The model under review builds one solid part; all positions refer to its coordinate system, in mm. A direction names the side the tool comes from. Round coordinates to 2 decimals unless told otherwise and drop trailing zeros. Order: outer loops, then holes, each group sorted by start corner. A loop starts at its lowest first (then second) coordinate and runs counter-clockwise, first axis right, second up. Notation, with made-up numbers: (73.25, 4) -> (97.25, 4) arc R27 cw to (97.25, 31) -> close; hole circle Ø9 at (-39.5, 10). An arc over 180 degrees is marked (long way). Use a Markdown table: item, result. Add a question column.
```python
from build123d import *

# Parameters (mm, degrees)
F0_W         = 34.544
F0_H         = 34.544
F1_DEPTH     = 38.1
F3_R         = 15.748
F4_R         = 2.286
F5_DEPTH     = 34.545
F6_R         = 4.445
F7_DEPTH     = 27.94
F8_S5_R      = 4.445
F8_T6_DEPTH  = 8
F8_S11_R     = 4.445
F8_T12_DEPTH = 8
F9_DEPTH     = 16.51
F2_R         = 8.4455
F10_DEPTH    = 33.782
F10_TAPER    = 0.8
F11_R        = 2.54
F12_R        = 3.81
F13_R        = 5.08
F15_DEPTH    = 38.101


# Not quite as in the source:
# - a fillet or chamfer that OpenCascade refuses, or shapes differently, is made with other operations: its cross-section is extruded or revolved along the edge and cut away or added


with BuildPart() as f1:
    # F0 (on Top) → F1 (new body)
    with BuildSketch(Plane.XY):
        with Locations((17.272, -17.272)):
            Rectangle(F0_W, F0_H)
    extrude(amount=F1_DEPTH)

    # F3
    f3_edges = [f1.edges().sort_by_distance(p)[0] for p in [
        (34.544, -34.544, 19.05),
        (34.544, 0, 19.05),
    ]]
    fillet(f3_edges, radius=F3_R)

    # F4 (on face) → F5 (cut, through all)
    with BuildSketch(Plane(origin=(0, 0, 0), x_dir=(0, -1, 0), z_dir=(-1, 0, 0))):
        with Locations((17.272, 10.16)):
            Circle(F4_R)
        with Locations((17.272, 27.94)):
            Circle(F4_R)
    extrude(amount=-F5_DEPTH, mode=Mode.SUBTRACT)

    # F6 (on face) → F7 (cut)
    with BuildSketch(Plane.YZ.offset(34.544)):
        with Locations((-17.272, 27.94)):
            Circle(F6_R)
        with Locations((-17.272, 10.16)):
            Circle(F6_R)
    extrude(amount=-F7_DEPTH, mode=Mode.SUBTRACT)

    # F8: chamfer of 2.54 on 2 edges, made by hand


with BuildPart() as f8_tool2:
    # F8_s3 → F8_t4 (revolve)
    with BuildSketch(Plane.XY.offset(27.94)):
        Polygon((4.064, -19.558), (6.604, -22.098), (6.604, -19.558), align=None)
    revolve(axis=Axis((6.604, -17.272, 27.94), (-1, 0, 0)))

    # F8_s5 → F8_t6 (intersect, symmetric)
    with BuildSketch(Plane.YZ.offset(5.3)):
        with Locations((-17.272, 27.94)):
            Circle(F8_S5_R)
    extrude(amount=F8_T6_DEPTH, both=True, mode=Mode.INTERSECT)


with BuildPart() as f1_1:
    add(f1.part)

    # F8_t1: cut F8_tool2
    add(f8_tool2.part, mode=Mode.SUBTRACT)


with BuildPart() as f8_tool8:
    # F8_s9 → F8_t10 (revolve)
    with BuildSketch(Plane.XY.offset(10.16)):
        Polygon((4.064, -19.558), (6.604, -22.098), (6.604, -19.558), align=None)
    revolve(axis=Axis((6.604, -17.272, 10.16), (-1, 0, 0)))

    # F8_s11 → F8_t12 (intersect, symmetric)
    with BuildSketch(Plane.YZ.offset(5.3)):
        with Locations((-17.272, 10.16)):
            Circle(F8_S11_R)
    extrude(amount=F8_T12_DEPTH, both=True, mode=Mode.INTERSECT)


with BuildPart() as f1_2:
    add(f1_1.part)

    # F8_t7: cut F8_tool8
    add(f8_tool8.part, mode=Mode.SUBTRACT)

    # F9 (add): a face of the model
    f9_faces = [f1_2.faces().sort_by_distance(p)[0] for p in [
        (0, -17.272, 19.05),
    ]]
    extrude(f9_faces, amount=F9_DEPTH)

    # F2 (on face) → F10 (join)
    with BuildSketch(Plane.XY.offset(38.1)):
        with Locations((17.272, -17.272)):
            Circle(F2_R)
    extrude(amount=F10_DEPTH, taper=F10_TAPER)

    # F11
    f11_edges = [f1_2.edges().sort_by_distance(p)[0] for p in [
        (1.143, 0, 38.1),
        (-16.51, -17.272, 38.1),
        (29.931518, -4.612482, 38.1),
        (1.143, -34.544, 38.1),
        (34.544, -17.272, 38.1),
        (29.931518, -29.931518, 38.1),
        (8.8265, -17.272, 38.1),
    ]]
    fillet(f11_edges, radius=F11_R)

    # F12
    f12_edges = [f1_2.edges().sort_by_distance(p)[0] for p in [
        (1.143, 0, 0),
        (-16.51, -17.272, 0),
        (1.143, -34.544, 0),
        (29.931518, -29.931518, 0),
        (34.544, -17.272, 0),
        (29.931518, -4.612482, 0),
    ]]
    fillet(f12_edges, radius=F12_R)

    # F13
    f13_edges = [f1_2.edges().sort_by_distance(p)[0] for p in [
        (9.298216, -17.272, 71.882),
    ]]
    fillet(f13_edges, radius=F13_R)

    # F14 (on face) → F15 (cut, through all)
    with BuildSketch(Plane.XY.offset(38.1)):
        with BuildLine():
            ThreePointArc((-6.6983271655, -3.81), (-8.9482084501, -5.1711725294), (-8.7866908377, -7.7957998383))
            Line((-8.7866908377, -7.7957998383), (-5.8592190016, -12.0243421801))
            ThreePointArc((-5.8592190016, -12.0243421801), (-3.7708553294, -13.1185423418), (-1.6824916571, -12.0243421801))
            Line((-1.6824916571, -12.0243421801), (1.244980179, -7.7957998383))
            ThreePointArc((1.244980179, -7.7957998383), (1.4064977914, -5.1711725294), (-0.8433834932, -3.81))
            Line((-0.8433834932, -3.81), (-6.6983271655, -3.81))
        make_face()
        with BuildLine():
            ThreePointArc((-1.6824916571, -22.5196578199), (-3.7708553294, -21.4254576582), (-5.8592190016, -22.5196578199))
            Line((-5.8592190016, -22.5196578199), (-8.7866908377, -26.7482001617))
            ThreePointArc((-8.7866908377, -26.7482001617), (-8.9482084501, -29.3728274706), (-6.6983271655, -30.734))
            Line((-6.6983271655, -30.734), (-0.8433834932, -30.734))
            ThreePointArc((-0.8433834932, -30.734), (1.4064977914, -29.3728274706), (1.244980179, -26.7482001617))
            Line((1.244980179, -26.7482001617), (-1.6824916571, -22.5196578199))
        make_face()
    extrude(amount=-F15_DEPTH, mode=Mode.SUBTRACT)


solid = f1_2.part
```
Q1. Add section A-A (z = 15.5). Write out the cut boundary in (x, y).
Q2. Add section D-D (z = 51). Write out the cut boundary in (x, y).
Q3. Add section B-B (z = 27.94). Write out the cut boundary in (x, y).
Q4. Machinability: for faces 1 (the flat face through (1, 0, 19)), 2 (the flat face through (4, -17, 38.1)), 3 (the flat face through (-7.343, -9.88, 19.317)), which of the approach directions +Z, -Z, +X, -X, +Y, -Y give a long, thin tool a straight path to every point of the face, cutting with its end or side? Answer none if there is none.
Q5. Wall thickness on line 1 (Y direction, x = -5.5, z = 33.5); line 2 (Z direction, x = 18, y = -16); line 3 (Z direction, x = 30, y = -19): over which ranges is each line inside the solid? List them lowest first. Write a range as [from, to].
Q6. Mouldability with a two-part tool opening along Y and no side actions: class faces 4 (the cylindrical face through (1.424, -5.206, 19.317)), 5 (the flat face through (-4, -30.734, 19)), 6 (the cylindrical face through (-15.786, -17.03, 37.336)), 7 (the cylindrical face through (0.9, -33.4, 1.09)) as pulls with the +Y half, pulls with the -Y half, needs draft (parallel to the pull), parting line crosses it, or undercut.
Q7. Insertion check: pin 1 (8 mm diameter, centred on y = -17.272, z = 27.94, fed in from +X); pin 2 (2 mm diameter, centred on y = -9.5, z = 28.5, fed in from +X); pin 3 (3 mm diameter, centred on y = -22, z = 42.5, fed in from +X). Each pin has a flat end and moves straight along its axis. Give the tip position at first contact, or say it passes through.
Q8. Add section C-C (x = 22). State how many separate pieces and enclosed holes the cut face has, then the cut area to 3 significant figures.
Report:
| question | item | result |
|---|---|---|
| 1 | outline | (-16.51, -34.54) -> (18.8, -34.54) arc R15.75 ccw to (34.54, -18.8) -> (34.54, -15.75) arc R15.75 ccw to (18.8, 0) -> (-16.51, 0) -> close; hole (-8.79, -26.75) arc R2.54 ccw to (-6.7, -30.73) -> (-0.84, -30.73) arc R2.54 ccw to (1.24, -26.75) -> (-1.68, -22.52) arc R2.54 ccw to (-5.86, -22.52) -> close; hole (-8.79, -7.8) -> (-5.86, -12.02) arc R2.54 ccw to (-1.68, -12.02) -> (1.24, -7.8) arc R2.54 ccw to (-0.84, -3.81) -> (-6.7, -3.81) arc R2.54 ccw to start |
| 2 | outline | circle Ø16.53 at (17.27, -17.27) |
| 3 | outline | (-16.51, -34.54) -> (18.8, -34.54) arc R15.75 ccw to (34.27, -21.72) -> (6.22, -21.72) -> (4.06, -19.56) -> (-16.51, -19.56) -> close; (-16.51, -14.99) -> (4.06, -14.99) -> (6.22, -12.83) -> (34.27, -12.83) arc R15.75 ccw to (18.8, 0) -> (-16.51, 0) -> close; hole (-8.79, -26.75) arc R2.54 ccw to (-6.7, -30.73) -> (-0.84, -30.73) arc R2.54 ccw to (1.24, -26.75) -> (-1.68, -22.52) arc R2.54 ccw to (-5.86, -22.52) -> close; hole (-8.79, -7.8) -> (-5.86, -12.02) arc R2.54 ccw to (-1.68, -12.02) -> (1.24, -7.8) arc R2.54 ccw to (-0.84, -3.81) -> (-6.7, -3.81) arc R2.54 ccw to start |
| 4 | face 1 | +Z, -Z, +X, -X, +Y |
| 4 | face 2 | +Z |
| 4 | face 3 | +Z, -Z |
| 5 | line 1 | y = [-34.54, -30.73], [-22.1, -12.44], [-3.81, 0] |
| 5 | line 2 | z = [0, 5.9], [14.42, 23.68], [32.2, 71.88] |
| 5 | line 3 | z = [0, 6.06], [14.26, 23.84], [32.04, 38.1] |
| 6 | face 4 | undercut |
| 6 | face 5 | undercut |
| 6 | face 6 | needs draft |
| 6 | face 7 | pulls with the -Y half |
| 7 | pin 1 | stops at x = 5.78 |
| 7 | pin 2 | stops at x = 33.64 |
| 7 | pin 3 | stops at x = 25.01 |
| 8 | separate pieces | 1 |
| 8 | enclosed holes | 2 |
| 8 | area | 1,600 mm² |
